from build123d import *

# Parameters (mm, degrees)
F0_R     = 12.5
F1_DEPTH = 0.5
F2_R     = 10
F3_DEPTH = 1
F4_R     = 10.75
F4_R_2   = 10
F5_DEPTH = 0.5


with BuildPart() as f1:
    # F0 (on Top) → F1 (new body)
    with BuildSketch(Plane.XY):
        Circle(F0_R)
    extrude(amount=F1_DEPTH)

    # F2 (on face) → F3 (join)
    with BuildSketch(Plane.XY.offset(0.5)):
        Circle(F2_R)
    extrude(amount=F3_DEPTH)

    # F4 (on face) → F5 (join)
    with BuildSketch(Plane.XY.offset(1.5)):
        Circle(F4_R)
        Circle(F4_R_2, mode=Mode.SUBTRACT)
        Circle(F4_R_2)
    extrude(amount=F5_DEPTH)

    # F6 (on Front) → F7 (revolve, cut)
    with BuildSketch(Plane.XZ):
        Polygon((-10.8236325905, 1.4508630848), (-10.0277131423, 1.4709283132), (-10.8236325905, 1.9524930976), align=None)
    revolve(axis=Axis((0, 0, 2.0342625212), (0, 0, 1)), mode=Mode.SUBTRACT)


solid = f1.part
Read the model definition and answer for the solid it produces. Units are mm, in the model's axes. A direction names the side the tool comes from. Coordinates: 2 decimals unless noted, no trailing zeros. Loops run counter-clockwise (first coordinate to the right, second up) from the corner with the lowest first, then second, coordinate; pieces in that order, holes last.
Q1. This flat-tipped pin is pushed along its axis until it touches: pin 1 Ø1 at (x, z) = (5.5, 1.5) entering from -Y. Where does it stop, or does it pass through?
Q2. Which of the six approach directions +Z, -Z, +X, -X, +Y, -Y give full straight-line access (tool end or side, diameter ignored) to faces 1 (the face through (-2.17, -9.76, 0.99)), 2 (the face through (0, 0, 2))?
Q3. The part is cut by section A-A on x = 0. Write down the section's boundary in (y, z), and give its area (3 significant figures).
Q4. Consider probe 1 along Z at (x, y) = (-10.5, -4.25); probe 2 along X at (y, z) = (0.25, 0.95); probe 3 along X at (y, z) = (3.25, 0.8). Determine where each line is inside the solid, lowest interval first.
Results below:
1. pin 1: stops at y = -9.4
2. face 1: none
2. face 2: +Z, +X, -X, +Y, -Y
3. outline: (-12.5, 0) - (12.5, 0) - (12.5, 0.5) - (10, 0.5) - (10, 1.5) - (10.08, 1.5) - (10.75, 1.91) - (10.75, 2) - (-10.75, 2) - (-10.75, 1.91) - (-10.08, 1.5) - (-10, 1.5) - (-10, 0.5) - (-12.5, 0.5) - close
3. area: 43.0 mm2
4. probe 1: z = 0 to 0.5
4. probe 2: x = -10 to 10
4. probe 3: x = -9.46 to 9.46
